Drawing for the job (mm, zero at the part's lowest x, y, z). A direction names the side the tool comes from. Coordinates: 2 decimals unless noted, no trailing zeros. Write each loop counter-clockwise with the first axis right and the second up, starting at its lowest first coordinate (ties: lowest second). Pieces come first, ordered by that corner, then holes. Notation, with made-up numbers: (24.25, -39.75) - (80.25, -39.75) arc R21 cw to (80.25, -1.75) - close; hole circle Ø3 at (44.5, 71). An arc over 180 degrees is marked (long way). Write each question's results on one line, items separated by ' | '.
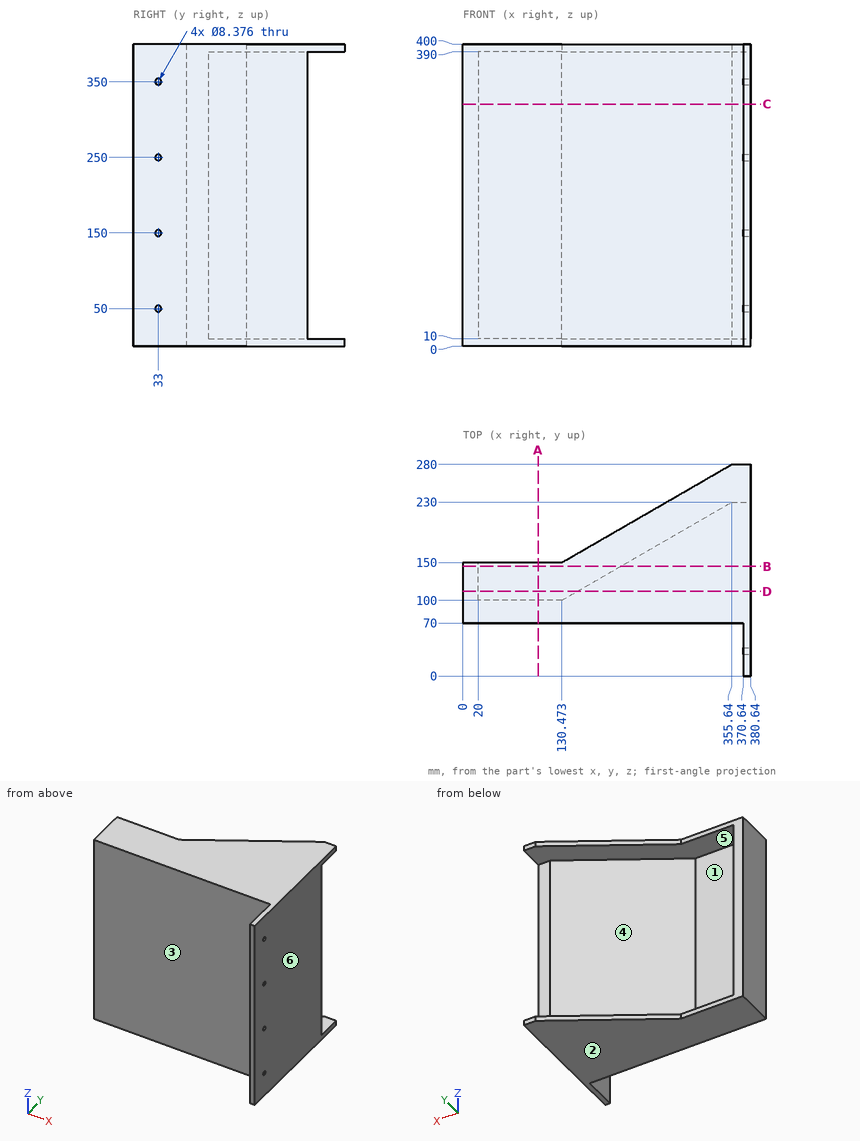
(1) Wall check: line 1 (Z direction, x = 378, y = 33); line 2 (Y direction, x = 377.5, z = 250); line 3 (X direction, y = 52, z = 154.5). Give the ranges that are in metal, low to high. Write a range as from..to.
Return value:
line 1: z = 0..45.81, 54.19..145.81, 154.19..245.81, 254.19..345.81, 354.19..400 | line 2: y = 0..28.81, 37.19..230 | line 3: x = 370.64..380.64
(2) 3-axis set-ups, long thin cutter, end or side, ignore diameter. For the marked faces 1 and 2: which of +Z, -Z, +X, -X, +Y, -Y reach the whole face in a straight line?
Return value:
face 1: +Y | face 2: -Z, +X, -X, +Y, -Y
(3) Saw through at A-A on x = 99.5. Write the cut outline in (y, z), then the cut area to 3 significant figures.
Return value:
outline: (70, 0) - (150, 0) - (150, 10) - (100, 10) - (100, 390) - (150, 390) - (150, 400) - (70, 400) - close | area: 13,000 mm^2
(4) Two-plate mould, pull along X, no slides. Class the marked faces 3, 4, 5 and 6: released by +X, released by -X, zero draft, split by the parting line, or undercut.
Return value:
face 3: zero draft | face 4: undercut | face 5: undercut | face 6: released by +X
(5) Saw through at B-B on y = 145. Write the cut outline in (x, z) (1 decimal), then the cut area to 3 significant figures.
Return value:
outline: (0, 0) - (380.6, 0) - (380.6, 400) - (0, 400) - close; hole (20, 10) - (208.4, 10) - (208.4, 390) - (20, 390) - close | area: 80,700 mm^2
(6) Saw through at D-D on y = 112. Write the cut outline in (x, z), then the cut area to 3 significant figures.
Return value:
outline: (0, 0) - (380.64, 0) - (380.64, 400) - (0, 400) - close; hole (20, 10) - (151.26, 10) - (151.26, 390) - (20, 390) - close | area: 102,000 mm^2
(7) Flat gauge pins, fed straight in: P1, Ø5, axis at y = 33, z = 50, coming from the +X side; P2, Ø6, axis at x = 254.5, z = 246, coming from the -Y side; P3, Ø10, axis at x = 328, z = 228.5, coming from the +Y side; P4, Ø9.5, axis at y = 33, z = 250, coming from the -X side. Where does each tip first touch, or does it go through?
Return value:
P1: passes through | P2: stops at y = 70 | P3: stops at y = 216.93 | P4: stops at x = 370.64
(8) Saw through at C-C on z = 320.5. Write the cut outline in (x, y).
Return value:
outline: (0, 70) - (370.64, 70) - (370.64, 0) - (380.64, 0) - (380.64, 230) - (355.64, 230) - (130.47, 100) - (20, 100) - (20, 150) - (0, 150) - close
